The listing builds one solid part. Answer for the finished solid, in the listing's coordinates (mm). A direction names the side the tool comes from. Coordinates: 2 decimals unless noted, no trailing zeros. Write each loop counter-clockwise with the first axis right and the second up, starting at its lowest first coordinate (ties: lowest second). Pieces come first, ordered by that corner, then holes.
from build123d import *

# Parameters (mm, degrees)
SKETCH1_W           = 15.8242
SKETCH1_H           = 15.8242
BOSS_EXTRUDE1_DEPTH = 9.5758
SKETCH2_W           = 13.4366
SKETCH2_H           = 13.4366
SKETCH2_R           = 3.2131
CUT_EXTRUDE1_DEPTH  = 8.4328
SKETCH3_R           = 2.4384
CUT_EXTRUDE2_DEPTH  = 8.4328
SKETCH4_R           = 2.4384
BOSS_EXTRUDE2_DEPTH = 1.9304
CIRPATTERN1_COUNT   = 4


with BuildPart() as part:
    # Sketch1 → Boss-Extrude1 (new body)
    with BuildSketch(Plane.XY):
        Rectangle(SKETCH1_W, SKETCH1_H)
    extrude(amount=BOSS_EXTRUDE1_DEPTH)

    # Sketch2 → Cut-Extrude1 (cut)
    with BuildSketch(Plane(origin=(0, 0, 0), x_dir=(-1, 0, 0), z_dir=(0, 0, -1))):
        Rectangle(SKETCH2_W, SKETCH2_H)
        Circle(SKETCH2_R, mode=Mode.SUBTRACT)
    extrude(amount=-CUT_EXTRUDE1_DEPTH, mode=Mode.SUBTRACT)

    # Sketch3 → Cut-Extrude2 (cut)
    with BuildSketch(Plane(origin=(0, 0, 0), x_dir=(-1, 0, 0), z_dir=(0, 0, -1))):
        Circle(SKETCH3_R)
    extrude(amount=-CUT_EXTRUDE2_DEPTH, mode=Mode.SUBTRACT)

    # Sketch4 → Boss-Extrude2 (add)
    with BuildSketch(Plane.XY.offset(9.5758)):
        with Locations((3.996213974, -3.996213974)):
            Circle(SKETCH4_R)
    boss_extrude2 = extrude(amount=BOSS_EXTRUDE2_DEPTH)

    # CirPattern1: Boss-Extrude2 ×4 about axis
    cirpattern1_axis = Axis((0, 0, 0), (0, 0, 1))
    for i in range(1, CIRPATTERN1_COUNT):
        add(boss_extrude2.rotate(cirpattern1_axis, i * 360 / CIRPATTERN1_COUNT))


solid = part.part
1. Section A-A on z = 4.5 is taken. Give the vertices of the cut face in (x, y).
Results found:
outline: (-7.91, -7.91) - (7.91, -7.91) - (7.91, 7.91) - (-7.91, 7.91) - close; circle Ø6.43 at (0, 0); hole (-6.72, -6.72) - (6.72, -6.72) - (6.72, 6.72) - (-6.72, 6.72) - close; hole circle Ø4.88 at (0, 0)
2. For a pull along Y with two mould halves and no side action, classify faces 4 (the flat face through (0, 7.912, 5)), 5 (the flat face through (-7.912, 0, 5)), 6 (the flat face through (-6.718, 0, 4)), 7 (the cylindrical face through (-2.326, 0.732, 4.157)) as pulls with the +Y half, pulls with the -Y half, needs draft (parallel to the pull), parting line crosses it, or undercut.
Results found:
face 4: pulls with the +Y half
face 5: needs draft
face 6: undercut
face 7: undercut
3. Section B-B on y = 0 is taken. Give the vertices of the cut face in (x, z), then the cut area to 3 significant figures.
Results found:
outline: (-7.91, 0) - (-6.72, 0) - (-6.72, 8.43) - (-3.21, 8.43) - (-3.21, 0) - (-2.44, 0) - (-2.44, 8.43) - (2.44, 8.43) - (2.44, 0) - (3.21, 0) - (3.21, 8.43) - (6.72, 8.43) - (6.72, 0) - (7.91, 0) - (7.91, 9.58) - (-7.91, 9.58) - close
area: 51.3 mm2
4. Find the intervals of material crossed by L1, parallel to Y at x = 0, z = 5; L2, parallel to X at y = 5, z = 2.75; L3, parallel to Y at x = -1, z = 2.5, in increasing order.
Results found:
L1: y = -7.91 to -6.72, -3.21 to -2.44, 2.44 to 3.21, 6.72 to 7.91
L2: x = -7.91 to -6.72, 6.72 to 7.91
L3: y = -7.91 to -6.72, -3.05 to -2.22, 2.22 to 3.05, 6.72 to 7.91
5. Flat-ended cylindrical pins translate along their axes: P1, Ø2, axis at x = -0.5, y = 6, coming from the +Z side; P2, Ø2.5, axis at x = 0.5, y = 0, coming from the -Z side. Find the tip coordinate at first contact, or state that the pin passes through.
Results found:
P1: stops at z = 9.58
P2: stops at z = 8.43
6. A tool of negligible diameter and unlimited length cuts with its end or side. For faces 1 (the flat face through (6.718, 0, 4)), 2 (the flat face through (-4, -4, 11.506)), 3 (the cylindrical face through (6.32, -3.26, 10.53)), from which of +Z, -Z, +X, -X, +Y, -Y can it reach the whole face along a straight path? Write none if from no direction.
Results found:
face 1: -Z
face 2: +Z, +X, -X, +Y, -Y
face 3: +Z
